Could you check a few things on this model? Use its own coordinates, in mm. A direction names the side the tool comes from. Give positions to 0.01 mm unless a question says otherwise; leave off trailing zeros. Loops run counter-clockwise (first coordinate to the right, second up) from the corner with the lowest first, then second, coordinate; pieces in that order, holes last. Notation, with made-up numbers: M 51.25,-15.5 L 77.25,-15.5 A20 ccw 77.25,23.5 Z; hole C 87.25,85.5 d7. An arc over 180 degrees is marked long. Answer in a Markdown table with one row per item. Add a question column.
Autodesk Inventor part; units mm, degrees
ref_plane "YZ Plane" through (0, 0, 0) normal (1, 0, 0) x (0, 1, 0)
ref_plane "XZ Plane" through (0, 0, 0) normal (0, 1, 0) x (-1, 0, 0)
ref_plane "XY Plane" through (0, 0, 0) normal (0, 0, 1) x (1, 0, 0)
sketch "Sketch1" plane through (0, 0, 0) normal (0, 1, 0) x (-1, 0, 0)
  circle A0 centre (0, 0) radius 2
  dimension "d0" = 4
extrude "Extrusion1" add sketch "Sketch1" along normal blind 20
sketch "Sketch2" plane through (0, 20, 0) normal (0, 1, 0) x (1, 0, 0)
  circle A0 centre (0, 0) radius 2
  circle A1 centre (0, 0) radius 3.5
  dimension "d3" = 7
extrude "Extrusion2" add sketch "Sketch2" along normal blind 4 contours A0 | A1
sketch "Sketch3" plane through (0, 24, 0) normal (0, 1, 0) x (1, 0, 0)
  circle A0 centre (0, 0) radius 3.5
  line L0 (0, 1.8475) -> (1.6, 0.9238)
  line L1 (1.6, 0.9238) -> (1.6, -0.9238)
  line L2 (1.6, -0.9238) -> (0, -1.8475)
  line L3 (0, -1.8475) -> (-1.6, -0.9238)
  line L4 (-1.6, -0.9238) -> (-1.6, 0.9238)
  line L5 (-1.6, 0.9238) -> (0, 1.8475)
  dimension "d6" = 1.6
extrude "Extrusion3" cut sketch "Sketch3" against normal blind 3 contours L0 L1 L2 L3 L4 L5
thread "Thread1"
chamfer "Chamfer1" distance 0.25 angle 45 1 edges at (2, 0, 0)
properties part number "M4x20SHCS"
Item 1: For faces 4 (the face through (-2, 24, 0)), 5 (the face through (0, 21, 0)), which set-ups out of +Z, -Z, +X, -X, +Y, -Y let a thin tool reach every point of the face, with its end or its side?
Item 2: Suppose I cut it at B-B (z = 0). List the corners of the cut face in (x, y) for me.
Item 3: Suppose I cut it at A-A (y = 22). List the corners of the cut face in (x, z) for me, then the cut area to 3 significant figures.
Item 4: I need wall thicknesses on L1, parallel to Y at x = -0.75, z = -3; L2, parallel to Y at x = -1, z = -1; L3, parallel to X at y = 19.5, z = -0.5. Which ranges of each line are inside material? Lowest first, please.
Item 5: Suppose I cut it at D-D (x = -3). List the corners of the cut face in (y, z) for me, then the cut area to 3 significant figures.
Item 6: If we mould it in two halves opening along X, with no side actions, what happens to faces 1 (the face through (0, 10, 2)), 2 (the face through (2, 20, 2)), 3 (the face through (0.79, 22.52, -1.39))? For each: +X half, -X half, draft (parallel to the pull), parting line (faces both ways), or undercut.
Item 7: Suppose I cut it at C-C (y = 6.5). List the corners of the cut face in (x, z) for me.
Item 8: For P1, Ø2, axis at y = 22, z = -0.5, coming from the +X side; P2, Ø1.5, axis at x = -0.5, y = 15.5, coming from the -Z side; P3, Ø1.5, axis at x = -2.5, y = 6, coming from the -Z side; P4, Ø1.5, axis at x = -2, y = 7.5, coming from the -Z side, each with a flat end and sliding along its axis, tell me the tip position at first contact or that it passes through.
Values found:
| question | item | result |
|---|---|---|
| 1 | face 4 | +Z, -Z, +X, -X, +Y |
| 1 | face 5 | +Y |
| 2 | outline | M -3.5,20 L -2,20 L -2,0.25 L -1.75,0 L 1.75,0 L 2,0.25 L 2,20 L 3.5,20 L 3.5,24 L 1.6,24 L 1.6,21 L -1.6,21 L -1.6,24 L -3.5,24 Z |
| 3 | outline | C 0,0 d7; hole M -1.6,-0.92 L 0,-1.85 L 1.6,-0.92 L 1.6,0.92 L 0,1.85 L -1.6,0.92 Z |
| 3 | area | 29.6 mm² |
| 4 | L1 | 20 to 24 |
| 4 | L2 | 0 to 21 |
| 4 | L3 | -1.94 to 1.94 |
| 5 | outline | M 20,-1.8 L 24,-1.8 L 24,1.8 L 20,1.8 Z |
| 5 | area | 14.4 mm² |
| 6 | face 1 | parting line |
| 6 | face 2 | draft |
| 6 | face 3 | undercut |
| 7 | outline | C 0,0 d4 |
| 8 | P1 | x = 3.5 |
| 8 | P2 | z = -2 |
| 8 | P3 | z = -0.97 |
| 8 | P4 | z = -1.56 |
